Source: CAD feature listing. Evaluate the final solid. Frame: model axes, mm. A direction names the side the tool comes from. Coordinates: 2 decimals unless noted, no trailing zeros.
Item 1: Contact query for flat-ended pins moving along their axis: P1, Ø4, axis at x = 11, z = -8.5, coming from the +Y side; P2, Ø8, axis at y = 4.5, z = -1, coming from the +X side; P3, Ø5, axis at x = 8.5, z = -3, coming from the +Y side. Output: stop coordinate, or through.
Item 2: Mould query, pull axis X, two halves, no side actions, for faces 4 (the flat face through (11.58, 9.64, -3.89)), 5 (the flat face through (-4.46, 13.68, -3.89)), 6 (the flat face through (-11.57, 9.62, -3.89)). Classes: released by +X, released by -X, zero draft, split by the parting line, or undercut.
Item 3: Ray query, line 1 (Y direction, x = 0, z = -1.75) (3 decimals); line 2 (Z direction, x = -14, y = -5.5); line 3 (Y direction, x = 15, z = 1). Return the intervals inside material, ascending.
Item 4: Reachability of faces 1 (the flat face through (8.035, 12.744, -3.886)), 2 (the cylindrical face through (14.007, -7.118, -3.886)), 3 (the flat face through (0.99, -15.03, -3.89)) from +Z, -Z, +X, -X, +Y, -Y: full face, straight path, thin tool, end or side. Return the list, or none.
from build123d import *

# Parameters (mm, degrees)
CUT_EXTRUDE1_START = 1.4986
CUT_EXTRUDE1_DEPTH = 10.922
CIRPATTERN1_COUNT  = 20
SKETCH4_R          = 9.525
CUT_EXTRUDE2_DEPTH = 31.500831465


with BuildPart() as part:
    # Sketch2 → Revolve1 (revolve)
    with BuildSketch(Plane(origin=(0, 0, 0), x_dir=(0, 0, -1), z_dir=(1, 0, 0)), mode=Mode.PRIVATE) as revolve1_sk:
        with BuildLine():
            Line((-3.1877, 3.175), (11.1125, 3.175))
            Line((11.1125, 3.175), (11.1125, 19.05))
            Line((11.1125, 19.05), (10.26795, 19.05))
            ThreePointArc((10.26795, 19.05), (9.646555263, 18.316132165), (9.4234, 17.380773865))
            Line((9.4234, 17.380773865), (9.4234, 15.711547731))
            Line((9.4234, 15.711547731), (-1.4986, 15.711547731))
            Line((-1.4986, 15.711547731), (-1.4986, 17.380773865))
            ThreePointArc((-1.4986, 17.380773865), (-1.721755263, 18.316132165), (-2.34315, 19.05))
            Line((-2.34315, 19.05), (-3.1877, 19.05))
            Line((-3.1877, 19.05), (-3.1877, 11.8999))
            Line((-3.1877, 11.8999), (-3.1877, 3.175))
        make_face()
    revolve(revolve1_sk.sketch.rotate(Axis((0, 0, 11.1125), (0, 0, -1)), 90), axis=Axis((0, 0, 11.1125), (0, 0, -1)))

    # Sketch3 → Cut-Extrude1 (cut)
    with BuildSketch(Plane.XY.offset(CUT_EXTRUDE1_START)):
        with BuildLine():
            Line((-0.690489274, 14.3891), (0.690489274, 14.3891))
            Line((0.690489274, 14.3891), (1.2827, 15.6591))
            ThreePointArc((1.2827, 15.6591), (0, 15.711547731), (-1.2827, 15.6591))
            Line((-1.2827, 15.6591), (-0.690489274, 14.3891))
        make_face()
    cut_extrude1 = extrude(amount=-CUT_EXTRUDE1_DEPTH, mode=Mode.SUBTRACT)

    # CirPattern1: Cut-Extrude1 ×20 about axis
    cirpattern1_axis = Axis((0, 0, 0), (0, 0, 1))
    for i in range(1, CIRPATTERN1_COUNT):
        add(cut_extrude1.rotate(cirpattern1_axis, i * 360 / CIRPATTERN1_COUNT), mode=Mode.SUBTRACT)

    # Sketch4 → Cut-Extrude2 (cut, through all)
    with BuildSketch(Plane.XY.offset(3.1877)):
        Circle(SKETCH4_R)
    extrude(amount=-CUT_EXTRUDE2_DEPTH, mode=Mode.SUBTRACT)


solid = part.part
Answer list:
1. P1: stops at y = 16.19
1. P2: stops at x = 18.91
1. P3: stops at y = 14.5
2. face 4: released by +X
2. face 5: undercut
2. face 6: released by -X
3. line 1: y = -14.389 to -9.525, 9.525 to 14.389
3. line 2: z = -11.11 to -9.42, 1.5 to 3.19
3. line 3: y = -3.65 to -0.98, 0.98 to 3.65
4. face 1: +X
4. face 2: +X, -Y
4. face 3: -Y
